Check sheet for the modelled part. Datum: model origin and axes. Units: mm. A direction names the side the tool comes from. Coordinates: 2 decimals unless noted, no trailing zeros. Loops run counter-clockwise (first coordinate to the right, second up) from the corner with the lowest first, then second, coordinate; pieces in that order, holes last. Notation, with made-up numbers: (13.25, 43.25) - (70.25, 43.25) arc R18 cw to (70.25, 69.25) - close; hole circle Ø8 at (80.5, 36.5). An arc over 180 degrees is marked (long way). Use a Markdown table: item, result. Add a question column.
1) Sectioned sample at A-A, the plane y = 13.5. Enter the section's corners in (x, z), then the cut area to 3 significant figures.
2) Sectioned sample at C-C, the plane x = -94.5. Enter the section's corners in (y, z), then the cut area to 3 significant figures.
3) Sectioned sample at D-D, the plane x = 45.5. Enter the section's corners in (y, z).
4) Tool access check on faces 3 (the cylindrical face through (-75.6, 23.2, 31)), 4 (the cylindrical face through (68.646, 46.967, 34.528)). Record the directions out of +Z, -Z, +X, -X, +Y, -Y that give a thin tool (end or side, any length) a straight path to the whole face; none if there is none.
5) Draft check along Y on faces 1 (the flat face through (-26, -19, 36.5)), 2 (the cylindrical face through (-25.473, -40.859, 34.528)). Enter one of: pulls with the +Y half, pulls with the -Y half, needs draft (parallel to the pull), parting line crosses it, or undercut.
6) Sectioned sample at B-B, the plane z = 31.25. Enter the section's corners in (x, y).
7) Go/stop test with flat-tipped pins: P1, Ø2, axis at x = -13, z = 34, coming from the +Y side; P2, Ø6, axis at x = -91, y = 10.5, coming from the -Z side; P3, Ø1.5, axis at y = 18.5, z = 33.5, coming from the -X side; P4, Ø3, axis at x = -120, y = 0, coming from the -Z side. Record where each tip stops, or that it passes through.
8) Thickness scan on line 1 (Y direction, x = -78, z = 32.45); line 2 (Y direction, x = 120, z = 33.4); line 3 (Y direction, x = 24, z = 34.25). Record the ranges inside material, lowest first.
from build123d import *

# Parameters (mm, degrees)
SKETCH010_W             = 248
SKETCH010_H             = 160
PAD006_DEPTH            = 4
SKETCH013_R             = 55
SKETCH013_R_2           = 2.75
SKETCH013_R_3           = 1.75
SKETCH013_R_4           = 1.4
POCKET005_DEPTH         = 5
SKETCH050_W             = 2
SKETCH050_H             = 2
POCKET031_DEPTH         = 838.3229460599
CHAMFER_SIZE            = 2
POCKET037_DEPTH         = 5
CHAMFER034_SIZE         = 1.5
CHAMFER035_SIZE         = 2
SKETCH058_R             = 3
PAD024_DEPTH            = 3
SKETCH059_R             = 1.4
POCKET042_DEPTH         = 5
BODY005_PLACEMENT_ANGLE = 180


with BuildPart() as part:
    # Sketch010 → Pad006 (new body)
    with BuildSketch(Plane.XY):
        Rectangle(SKETCH010_W, SKETCH010_H)
    extrude(amount=PAD006_DEPTH)

    # Sketch013 (on Face6 of Pad006) → Pocket005 (cut)
    with BuildSketch(Plane.XY.offset(4)):
        with Locations((-25, -13.5)):
            Circle(SKETCH013_R)
        with Locations((-77.5, 39)):
            Circle(SKETCH013_R_2)
        with Locations((27.5, 39)):
            Circle(SKETCH013_R_2)
        with Locations((27.5, -66)):
            Circle(SKETCH013_R_2)
        with Locations((-77.5, -66)):
            Circle(SKETCH013_R_2)
        with Locations((-50, 75)):
            Circle(SKETCH013_R_3)
        with Locations((90, -75)):
            Circle(SKETCH013_R_3)
        with Locations((-90, -75)):
            Circle(SKETCH013_R_3)
        with Locations((120, 65)):
            Circle(SKETCH013_R_3)
        with Locations((120, -65)):
            Circle(SKETCH013_R_3)
        with Locations((-120, 65)):
            Circle(SKETCH013_R_4)
        with Locations((-120, -65)):
            Circle(SKETCH013_R_4)
        with Locations((100, 30)):
            Circle(SKETCH013_R_3)
        with Locations((100, -30)):
            Circle(SKETCH013_R_3)
        with Locations((50, 75)):
            Circle(SKETCH013_R_3)
        with Locations((-120, 0)):
            Circle(SKETCH013_R_4)
        with Locations((120, 0)):
            Circle(SKETCH013_R_3)
    extrude(amount=-POCKET005_DEPTH, mode=Mode.SUBTRACT)

    # Sketch050 (on Face2 of Pocket005) → Pocket031 (cut, through all)
    with BuildSketch(Plane(origin=(-124, 0, 0), x_dir=(0, -1, 0), z_dir=(-1, 0, 0))):
        with Locations((79, 1)):
            Rectangle(SKETCH050_W, SKETCH050_H)
    pocket031 = extrude(amount=-POCKET031_DEPTH, mode=Mode.SUBTRACT)

    # Mirrored004: Pocket031 across Sketch050 V_Axis
    add(pocket031.mirror(Plane(origin=(-124, 0, 0), x_dir=(-1, 0, 0), z_dir=(0, -1, 0))), mode=Mode.SUBTRACT)

    # Chamfer
    chamfer_edges = [part.edges().sort_by_distance(p)[0] for p in [
        (-124, 0, 0),
    ]]
    chamfer(chamfer_edges, length=CHAMFER_SIZE)

    # Sketch051 → Pocket037 (cut)
    with BuildSketch(Plane(origin=(0, 0, 0), x_dir=(1, 0, 0), z_dir=(0, 0, -1))):
        Polygon((-125, 75.7573593129), (-120.7573593129, 80), (-125, 80), align=None)
        Polygon((-120.7573593129, -80), (-125, -75.7573593129), (-125, -80), align=None)
    extrude(amount=-POCKET037_DEPTH, mode=Mode.SUBTRACT)

    # Chamfer034
    chamfer034_edges = [part.edges().sort_by_distance(p)[0] for p in [
        (124, -80, 3),
        (124, 80, 3),
    ]]
    chamfer(chamfer034_edges, length=CHAMFER034_SIZE)

    # Chamfer035
    chamfer035_edges = [part.edges().sort_by_distance(p)[0] for p in [
        (124, 0, 0),
    ]]
    chamfer(chamfer035_edges, length=CHAMFER035_SIZE)

    # Sketch058 (on Face9 of Chamfer035) → Pad024 (join)
    with BuildSketch(Plane(origin=(0, 0, 0), x_dir=(1, 0, 0), z_dir=(0, 0, -1))):
        with Locations((50, 25)):
            Circle(SKETCH058_R)
        with Locations((78, 25)):
            Circle(SKETCH058_R)
        with Locations((50, -25)):
            Circle(SKETCH058_R)
        with Locations((78, -25)):
            Circle(SKETCH058_R)
    extrude(amount=PAD024_DEPTH)

    # Sketch059 (on Face39 of Pad024) → Pocket042 (cut)
    with BuildSketch(Plane(origin=(0, 0, -3), x_dir=(1, 0, 0), z_dir=(0, 0, -1))):
        with Locations((50, 25)):
            Circle(SKETCH059_R)
        with Locations((78, 25)):
            Circle(SKETCH059_R)
        with Locations((50, -25)):
            Circle(SKETCH059_R)
        with Locations((78, -25)):
            Circle(SKETCH059_R)
    extrude(amount=-POCKET042_DEPTH, mode=Mode.SUBTRACT)


with BuildPart() as part_1:
    # Body005 placement: moved
    add(part.part.moved(Location((0, 0, 32.5))).rotate(Axis((0, 0, 32.5), (0, 0, 1)), BODY005_PLACEMENT_ANGLE))


solid = part_1.part
Solved:
| question | item | result |
|---|---|---|
| 1 | outline | (-124, 34.5) - (-122, 32.5) - (-30, 32.5) - (-30, 36.5) - (-124, 36.5) - close; (80, 32.5) - (122, 32.5) - (124, 34.5) - (124, 36.5) - (80, 36.5) - close |
| 1 | area | 548 mm2 |
| 2 | outline | (-80, 34.5) - (-78, 34.5) - (-78, 32.5) - (78, 32.5) - (78, 34.5) - (80, 34.5) - (80, 36.5) - (-80, 36.5) - close |
| 2 | area | 632 mm2 |
| 3 | outline | (-80, 34.5) - (-78, 34.5) - (-78, 32.5) - (-37.54, 32.5) - (-37.54, 36.5) - (-80, 36.5) - close; (64.54, 32.5) - (78, 32.5) - (78, 34.5) - (80, 34.5) - (80, 36.5) - (64.54, 36.5) - close |
| 4 | face 3 | -Z |
| 4 | face 4 | +Z, -Z |
| 5 | face 1 | needs draft |
| 5 | face 2 | undercut |
| 6 | outline | circle Ø6 at (-78, -25); circle Ø6 at (-78, 25); circle Ø6 at (-50, -25); circle Ø6 at (-50, 25); hole circle Ø2.8 at (-78, -25); hole circle Ø2.8 at (-78, 25); hole circle Ø2.8 at (-50, -25); hole circle Ø2.8 at (-50, 25) |
| 7 | P1 | stops at y = 80 |
| 7 | P2 | stops at z = 32.5 |
| 7 | P3 | stops at x = -123.75 |
| 7 | P4 | passes through |
| 8 | line 1 | y = -28 to -26.4, -23.6 to -22, 22 to 23.6, 26.4 to 28 |
| 8 | line 2 | y = -78 to -66.4, -63.6 to -1.4, 1.4 to 63.6, 66.4 to 78 |
| 8 | line 3 | y = -78 to -41.49, 68.49 to 78 |
